from build123d import *

# Parameters (mm, degrees)
SKETCH1_R           = 2
BOSS_EXTRUDE1_DEPTH = 28.5


with BuildPart() as part:
    # Sketch1 → Boss-Extrude1 (new, symmetric)
    with BuildSketch(Plane(origin=(0, 0, 0), x_dir=(0, 0, -1), z_dir=(1, 0, 0))):
        with BuildLine():
            Line((0, 0), (6, 0))
            ThreePointArc((6, 0), (11, 5), (6, 10))
            ThreePointArc((6, 10), (3.878679656, 10.878679656), (3, 13))
            Line((3, 13), (3, 39))
            ThreePointArc((3, 39), (3.878679656, 41.121320344), (6, 42))
            ThreePointArc((6, 42), (11, 47), (6, 52))
            Line((6, 52), (0, 52))
            Line((0, 52), (0, 0))
        make_face()
        with Locations(Location((6, 5, 0), (0, 0, 180))):
            Circle(SKETCH1_R, mode=Mode.SUBTRACT)
        with Locations(Location((6, 47, 0), (0, 0, 180))):
            Circle(SKETCH1_R, mode=Mode.SUBTRACT)
    extrude(amount=BOSS_EXTRUDE1_DEPTH, both=True)


solid = part.part
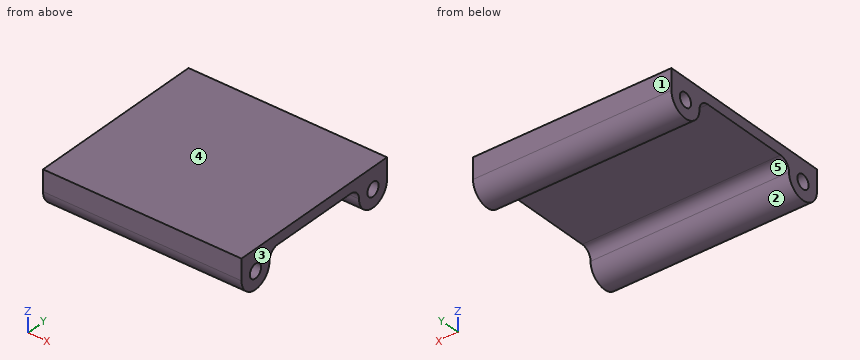
Geometry check sheet. Reference: the model listing, model coordinates, mm. Face numbers are marked on the shaded views. A direction names the side the tool comes from. Give positions to 0.01 mm unless a question says otherwise; leave off trailing zeros. Loops run counter-clockwise (first coordinate to the right, second up) from the corner with the lowest first, then second, coordinate; pieces in that order, holes last.
(1) Depth check by flat-ended pin: pin 1 Ø5 at (x, y) = (-2.5, 12) entering from -Z; pin 2 Ø5 at (x, y) = (-10, 35.5) entering from -Z; pin 3 Ø2.5 at (y, z) = (5, -6) entering from -X. Enter the tip coordinate at first touch or a pass-through.
From the geometry:
pin 1: stops at z = -8.18
pin 2: stops at z = -3
pin 3: passes through
(2) Section check A-A on y = 5. Record the cut outline in (x, z), then the cut area to 3 significant figures.
From the geometry:
outline: (-28.5, -11) - (28.5, -11) - (28.5, -8) - (-28.5, -8) - close; (-28.5, -4) - (28.5, -4) - (28.5, 0) - (-28.5, 0) - close
area: 399 mm2
(3) Set-up check for the marked faces 4 and 5: record each of +Z, -Z, +X, -X, +Y, -Y from which the full face is reachable in a straight line by a thin tool's end or side.
From the geometry:
face 4: +Z, +X, -X, +Y, -Y
face 5: -Z, +X, -X
(4) Release check for a two-part mould opening along Y. For the marked faces 1, 2 and 3 record: released by +Y, released by -Y, zero draft, split by the parting line, or undercut.
From the geometry:
face 1: released by +Y
face 2: undercut
face 3: zero draft
(5) Section check D-D on y = 19.5. Record the cut outline in (x, z).
From the geometry:
outline: (-28.5, -3) - (28.5, -3) - (28.5, 0) - (-28.5, 0) - close
(6) Section check C-C on x = 16. Record the cut outline in (y, z), then the cut area to 3 significant figures.
From the geometry:
outline: (0, -6) arc R5 ccw to (10, -6) arc R3 cw to (13, -3) - (39, -3) arc R3 cw to (42, -6) arc R5 ccw to (52, -6) - (52, 0) - (0, 0) - close; hole circle Ø4 at (5, -6); hole circle Ø4 at (47, -6)
area: 273 mm2
(7) Thickness scan on L1, parallel to Y at x = -5.5, z = -6; L2, parallel to Y at x = 6.5, z = -5.5; L3, parallel to Z at x = -6, y = 47. Record the ranges inside material, lowest first.
From the geometry:
L1: y = 0 to 3, 7 to 10, 42 to 45, 49 to 52
L2: y = 0 to 3.06, 6.94 to 10.04, 41.96 to 45.06, 48.94 to 52
L3: z = -11 to -8, -4 to 0
(8) Section check B-B on z = -9. Record the cut outline in (x, y).
From the geometry:
outline: (-28.5, 1) - (28.5, 1) - (28.5, 9) - (-28.5, 9) - close; (-28.5, 43) - (28.5, 43) - (28.5, 51) - (-28.5, 51) - close
